Design review of the part built by this model. Coordinates are the model's own, in mm. A direction names the side the tool comes from. Give positions to 0.01 mm unless a question says otherwise; leave off trailing zeros. Write each loop counter-clockwise with the first axis right and the second up, starting at its lowest first coordinate (ties: lowest second). Pieces come first, ordered by that corner, then holes.
```python
from build123d import *

# Parameters (mm, degrees)
SKETCH1_W                    = 82
SKETCH1_H                    = 725.7
BASE_FLANGE1_DEPTH           = 1
EDGE_FLANGE1_STRIP_W         = 6
EDGE_FLANGE1_STRIP_H         = 1
EDGE_FLANGE1_STRIP_CUT_DEPTH = 725.7
EDGE_FLANGE1_DEPTH           = 725.7
EDGE_FLANGE2_STRIP_W         = 6
EDGE_FLANGE2_STRIP_H         = 1
EDGE_FLANGE2_STRIP_CUT_DEPTH = 725.7
EDGE_FLANGE2_DEPTH           = 725.7
SKETCH19_R                   = 2.5
CUT_EXTRUDE2_DEPTH           = 10
CUT_EXTRUDE3_START           = -725.7
CUT_EXTRUDE3_DEPTH           = 20.5


# Read off the part's stored shape, not the designer's step: Cut-Extrude3
# Sheet-metal steps are written as plain solids
with BuildPart() as part:
    # Sketch1 → Base-Flange1 (new body)
    with BuildSketch(Plane(origin=(0, 0, 0), x_dir=(1, 0, 0), z_dir=(0, 1, 0))):
        with Locations((41, 362.85)):
            Rectangle(SKETCH1_W, SKETCH1_H)
    extrude(amount=-BASE_FLANGE1_DEPTH)

    # Edge-Flange1 strip (across the edge) → Edge-Flange1 strip cut (cut)
    with BuildSketch(Plane(origin=(82, 0, 0), x_dir=(-1, 0, 0), z_dir=(0, 0, -1))):
        with Locations((-1, -0.5)):
            Rectangle(EDGE_FLANGE1_STRIP_W, EDGE_FLANGE1_STRIP_H)
    extrude(amount=EDGE_FLANGE1_STRIP_CUT_DEPTH, mode=Mode.SUBTRACT)

    # Edge-Flange1 section (across the edge) → Edge-Flange1 (add)
    with BuildSketch(Plane(origin=(82, 0, 0), x_dir=(-1, 0, 0), z_dir=(0, 0, -1))):
        with BuildLine():
            Line((0, 1), (0, 19))
            Line((0, 19), (1, 19))
            Line((1, 19), (1, 1))
            ThreePointArc((1, 1), (1.292893219, 0.292893219), (2, 0))
            Line((2, 0), (2, -1))
            ThreePointArc((2, -1), (0.585786438, -0.414213562), (0, 1))
        make_face()
    extrude(amount=EDGE_FLANGE1_DEPTH)

    # Edge-Flange2 strip (across the edge) → Edge-Flange2 strip cut (cut)
    with BuildSketch(Plane(origin=(81, 19, 0), x_dir=(0, -1, 0), z_dir=(0, 0, -1))):
        with Locations((-1, -0.5)):
            Rectangle(EDGE_FLANGE2_STRIP_W, EDGE_FLANGE2_STRIP_H)
    extrude(amount=EDGE_FLANGE2_STRIP_CUT_DEPTH, mode=Mode.SUBTRACT)

    # Edge-Flange2 section (across the edge) → Edge-Flange2 (add)
    with BuildSketch(Plane(origin=(81, 19, 0), x_dir=(0, -1, 0), z_dir=(0, 0, -1))):
        with BuildLine():
            Line((0, 1), (0, 12))
            Line((0, 12), (1, 12))
            Line((1, 12), (1, 1))
            ThreePointArc((1, 1), (1.292893219, 0.292893219), (2, 0))
            Line((2, 0), (2, -1))
            ThreePointArc((2, -1), (0.585786438, -0.414213562), (0, 1))
        make_face()
    extrude(amount=EDGE_FLANGE2_DEPTH)

    # Sketch19 → Cut-Extrude2 (cut)
    with BuildSketch(Plane(origin=(0, 19, 0), x_dir=(1, 0, 0), z_dir=(0, 1, 0))):
        with Locations(Location((75, 63, 0), (0, 0, 180))):
            Circle(SKETCH19_R)
        with Locations(Location((75, 108, 0), (0, 0, 180))):
            Circle(SKETCH19_R)
        with Locations(Location((75, 276, 0), (0, 0, 180))):
            Circle(SKETCH19_R)
        with Locations(Location((75, 444, 0), (0, 0, 180))):
            Circle(SKETCH19_R)
        with Locations(Location((75, 612, 0), (0, 0, 180))):
            Circle(SKETCH19_R)
        with Locations((75, 780)):
            Circle(SKETCH19_R)
    extrude(amount=-CUT_EXTRUDE2_DEPTH, mode=Mode.SUBTRACT)

    # Cut-Extrude3 outline → Cut-Extrude3 (cut)
    with BuildSketch(Plane.XY.offset(CUT_EXTRUDE3_START)):
        with BuildLine():
            ThreePointArc((81, 1), (80.707106781, 0.292893219), (80, 0))
            Line((80, 0), (80, -1))
            ThreePointArc((80, -1), (81.414213562, -0.414213562), (82, 1))
            Line((82, 1), (82, 17))
            ThreePointArc((82, 17), (81.414213562, 18.414213562), (80, 19))
            Line((80, 19), (69, 19))
            Line((69, 19), (69, 18))
            Line((69, 18), (80, 18))
            ThreePointArc((80, 18), (80.707106781, 17.707106781), (81, 17))
            Line((81, 17), (81, 1))
        make_face()
    extrude(amount=CUT_EXTRUDE3_DEPTH, mode=Mode.SUBTRACT)


solid = part.part
```
(1) Tool access review of faces 1 (the face through (82, 9, -348)), 2 (the face through (81, 9, -348)): name each direction out of +Z, -Z, +X, -X, +Y, -Y from which nothing blocks a thin tool from reaching the whole face with its end or side.
Resolved:
face 1: +Z, -Z, +X, +Y, -Y
face 2: +Z, -Z, -X
(2) Consider section C-C, the plane x = 53. Give the boundary of the cut face in (y, z), then the cut area to 3 significant figures.
Resolved:
outline: (-1, -725.7) - (0, -725.7) - (0, 0) - (-1, 0) - close
area: 726 mm2
(3) Mouldability with a two-part tool opening along Y and no side actions: class faces 3 (the face through (39, -1, -368)), 4 (the face through (43.8, -0.7, 0)), 5 (the face through (75, 19, -348)), 6 (the face through (74, 18, -348)) as pulls with the +Y half, pulls with the -Y half, needs draft (parallel to the pull), parting line crosses it, or undercut.
Resolved:
face 3: pulls with the -Y half
face 4: needs draft
face 5: pulls with the +Y half
face 6: undercut
(4) To check wall thickness, follow L1, parallel to Z at x = 75, y = 18.3; L2, parallel to X at y = 18.7, z = -612; L3, parallel to X at y = 18.4, z = -444. State the ranges of each line that lie inside material, in increasing order.
Resolved:
L1: z = -705.2 to -614.5, -609.5 to -446.5, -441.5 to -278.5, -273.5 to -110.5, -105.5 to -65.5, -60.5 to 0
L2: x = 69 to 72.5, 77.5 to 81.05
L3: x = 69 to 72.5, 77.5 to 81.43
(5) Consider section B-B, the plane y = 7.25. Give the boundary of the cut face in (x, z), then the cut area to 3 significant figures.
Resolved:
outline: (81, -705.2) - (82, -705.2) - (82, 0) - (81, 0) - close
area: 705 mm2
(6) Consider section A-A, the plane z = -91.5. Give the boundary of the cut face in (x, y), then the cut area to 3 significant figures.
Resolved:
outline: (0, -1) - (80, -1) arc R2 ccw to (82, 1) - (82, 17) arc R2 ccw to (80, 19) - (69, 19) - (69, 18) - (80, 18) arc R1 cw to (81, 17) - (81, 1) arc R1 cw to (80, 0) - (0, 0) - close
area: 112 mm2
(7) Clearance check with flat-ended pins moving along their axes: P1, Ø2, axis at y = 2.5, z = -521, coming from the -X side; P2, Ø3, axis at x = 75, z = -108, coming from the +Y side; P3, Ø0.8, axis at y = -0.5, z = -711, coming from the +X side; P4, Ø6.5, axis at x = 76.5, y = 7, coming from the -Z side. State where each tip first meets the part, or that it passes through.
Resolved:
P1: stops at x = 81
P2: stops at y = 0
P3: stops at x = 80
P4: passes through
